Could you check a few things on this model? Use its own coordinates, in mm. Face numbers are marked on the shaded views. A direction names the side the tool comes from. Give positions to 0.01 mm unless a question says otherwise; leave off trailing zeros. Loops run counter-clockwise (first coordinate to the right, second up) from the corner with the lowest first, then second, coordinate; pieces in that order, holes last. Notation, with made-up numbers: (33, 18) - (76, 18) arc R17 cw to (76, 23) - close; hole circle Ø11 at (-34, -29). An arc over 180 degrees is marked (long way). Write each question's results on one line, items separated by ' | '. Start each with the question number.
1) I want a section at C-C, the plane x = 11.5. Write out the boundary of the cut face in (y, z).
2) I want a section at A-A, the plane z = 0. Write out the boundary of the cut face in (x, y), and give its area (3 significant figures).
3) If I drill on probe 1 along Y at (x, z) = (-10, 0); probe 2 along Y at (x, z) = (5.5, 0); probe 3 along X at (y, z) = (28, 79), over which ranges is the centre line in solid material (lowest first)? Write a range as [from, to].
4) I want a section at D-D, the plane z = 40. Write out the boundary of the cut face in (x, y), and give its area (3 significant figures).
5) I'm going to push flat-ended pins straight in: pin 1 (1 mm diameter, centred on x = 6, y = 25.5, fed in from -Z); pin 2 (5 mm diameter, centred on x = 0.5, y = -80, fed in from -Z); pin 3 (1.5 mm diameter, centred on x = -10, y = 6.5, fed in from +Z). Where does each tip first touch, or does it pass through?
6) On a 3-axis mill with a long thin cutter (end or side, diameter ignored), from which of +Z, -Z, +X, -X, +Y, -Y can I reach the whole of each face in a straight line? I mean the marked faces 1 and 2. Say none if no direction works.
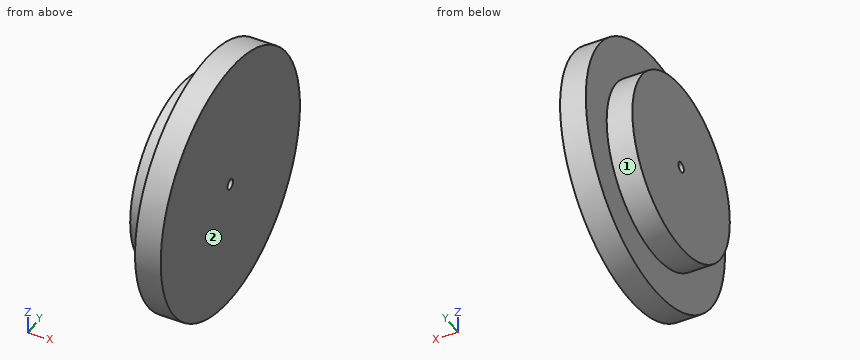
from build123d import *

# Parameters (mm, degrees)
SKETCH1_R           = 100
BOSS_EXTRUDE1_DEPTH = 20
SKETCH2_R           = 70
BOSS_EXTRUDE2_DEPTH = 20
CUT_EXTRUDE1_REACH  = 148.969
SKETCH3_R           = 4


with BuildPart() as part:
    # Sketch1 → Boss-Extrude1 (new body)
    with BuildSketch(Plane(origin=(0, 0, 0), x_dir=(0, 0, -1), z_dir=(1, 0, 0))):
        Circle(SKETCH1_R)
    extrude(amount=BOSS_EXTRUDE1_DEPTH)

    # Sketch2 → Boss-Extrude2 (add)
    with BuildSketch(Plane.ZY):
        Circle(SKETCH2_R)
    extrude(amount=BOSS_EXTRUDE2_DEPTH)

    # Sketch3 → Cut-Extrude1 (cut, up to next)
    with BuildSketch(Plane.ZY.offset(20), mode=Mode.PRIVATE) as cut_extrude1_sk1:
        Circle(SKETCH3_R)
    cut_extrude1_tool1 = extrude(cut_extrude1_sk1.sketch, amount=-CUT_EXTRUDE1_REACH, mode=Mode.PRIVATE) & part.part
    add(cut_extrude1_tool1.solids().sort_by_distance((-20, 0, 0))[0], mode=Mode.SUBTRACT)


solid = part.part
Answers:
1) outline: circle Ø200 at (0, 0); hole circle Ø8 at (0, 0)
2) outline: (-20, -70) - (0, -70) - (0, -100) - (20, -100) - (20, -4) - (-20, -4) - close; (-20, 4) - (20, 4) - (20, 100) - (0, 100) - (0, 70) - (-20, 70) - close | area: 6,480 mm2
3) probe 1: y = [-70, -4], [4, 70] | probe 2: y = [-100, -4], [4, 100] | probe 3: x = [0, 20]
4) outline: (-20, -57.45) - (0, -57.45) - (0, -91.65) - (20, -91.65) - (20, 91.65) - (0, 91.65) - (0, 57.45) - (-20, 57.45) - close | area: 5,960 mm2
5) pin 1: stops at z = -96.82 | pin 2: stops at z = -63.2 | pin 3: stops at z = 69.76
6) face 1: -X | face 2: +Z, -Z, +X, +Y, -Y
